Verification items for the finished model (mm, model axes). Round coordinates to 2 decimals unless told otherwise and drop trailing zeros. Order: outer loops, then holes, each group sorted by start corner. A loop starts at its lowest first (then second) coordinate and runs counter-clockwise, first axis right, second up. Notation, with made-up numbers: (57.25, 80) -> (108.25, 80) arc R18 cw to (108.25, 96) -> close; hole circle Ø10 at (10.5, 17.25). An arc over 180 degrees is marked (long way). Answer in a Markdown table with one row per item. Add a question column.
Autodesk Inventor part; units mm, degrees
ref_plane "YZ Plane" through (0, 0, 0) normal (1, 0, 0) x (0, 1, 0)
ref_plane "XZ Plane" through (0, 0, 0) normal (0, 1, 0) x (-1, 0, 0)
ref_plane "XY Plane" through (0, 0, 0) normal (0, 0, 1) x (1, 0, 0)
sketch "Szkic1" plane through (0, 0, 0) normal (0, 0, 1) x (1, 0, 0)
  line L0 (0, 0) -> (15.9, 0)
  line L1 (15.9, 0) -> (15.9, 1.5)
  line L2 (15.9, 1.5) -> (0, 1.5)
  line L3 (0, 1.5) -> (0, 0)
  dimension "d0" = 15.9
  dimension "d1" = 1.5
extrude "Wyciągnięcie proste1" add sketch "Szkic1" along normal mid plane 399
sketch "Szkic2" plane through (0, 0, 0) normal (0, 1, 0) x (-1, 0, 0)
  line L0 (0, -199.5) -> (-15.9, -199.5) construction
  line L1 (-7.95, -199.5) -> (-7.95, -178.6885) construction
  line L2 (-15.9, 199.5) -> (0, 199.5)
  point P0 (0, 0)
  point P1 (-7.95, -150)
  point P2 (-7.95, -60)
  point P3 (-7.95, 30)
  point P4 (-7.95, 150)
  dimension "d4" = 49.5
  dimension "d5" = 90
  dimension "d6" = 49.5
  dimension "d7" = 90
hole "Otwór1" at (7.95, 0, -150) at (7.95, 0, -60) at (7.95, 0, 30) at (7.95, 0, 150) direction (0, 1, 0) diameter 6 end through all
properties part number "Listwa_oparcia" material "Polistyren"
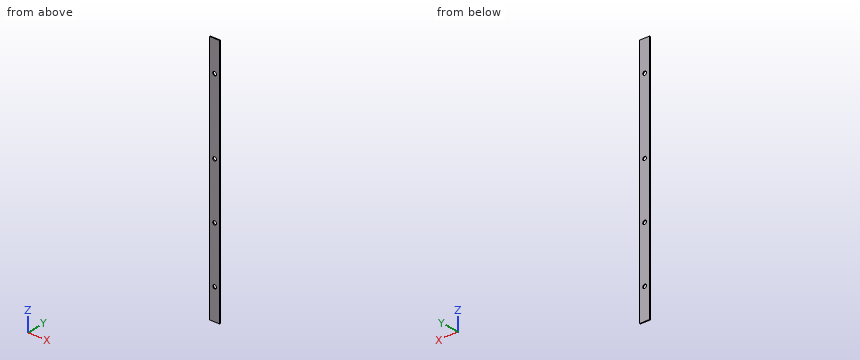
1) Cross-section at B-B, the plane y = 0.3. Record the boundary of the cut face in (x, z), and give its area (3 significant figures).
2) Thickness scan on L1, parallel to Z at x = 7.95, y = 0.45; L2, parallel to X at y = 0.8, z = -60; L3, parallel to Z at x = 5.75, y = 0.65. Record the ranges inside material, lowest first. Write a range as [from, to].
3) Cross-section at A-A, the plane x = 7.95. Record the boundary of the cut face in (y, z).
4) Depth check by flat-ended pin: P1, Ø3.5, axis at x = 7.95, z = -150, coming from the +Y side. Enter the tip coordinate at first touch or a pass-through.
Results below:
| question | item | result |
|---|---|---|
| 1 | outline | (0, -199.5) -> (15.9, -199.5) -> (15.9, 199.5) -> (0, 199.5) -> close; hole circle Ø6 at (7.95, -150); hole circle Ø6 at (7.95, -60); hole circle Ø6 at (7.95, 30); hole circle Ø6 at (7.95, 150) |
| 1 | area | 6,230 mm² |
| 2 | L1 | [-199.5, -153], [-147, -63], [-57, 27], [33, 147], [153, 199.5] |
| 2 | L2 | [0, 4.95], [10.95, 15.9] |
| 2 | L3 | [-199.5, -152.04], [-147.96, -62.04], [-57.96, 27.96], [32.04, 147.96], [152.04, 199.5] |
| 3 | outline | (0, -199.5) -> (1.5, -199.5) -> (1.5, -153) -> (0, -153) -> close; (0, -147) -> (1.5, -147) -> (1.5, -63) -> (0, -63) -> close; (0, -57) -> (1.5, -57) -> (1.5, 27) -> (0, 27) -> close; (0, 33) -> (1.5, 33) -> (1.5, 147) -> (0, 147) -> close; (0, 153) -> (1.5, 153) -> (1.5, 199.5) -> (0, 199.5) -> close |
| 4 | P1 | through |
